from build123d import *

# Parameters (mm, degrees)
BOX001_W               = 20
BOX001_H               = 7.071068
BOX001_DEPTH           = 7.071068
BOX001_PLACEMENT_ANGLE = 45
BOX_W                  = 20
BOX_H                  = 10
BOX_DEPTH              = 10


with BuildPart() as cube001:
    # Box001 → Box001 (new body)
    with BuildSketch(Plane.XY):
        with Locations((10, 3.535534)):
            Rectangle(BOX001_W, BOX001_H)
    extrude(amount=BOX001_DEPTH)


with BuildPart() as cube001_1:
    # Box001 placement: moved
    add(cube001.part.moved(Location((0, 5, 5))).rotate(Axis((0, 5, 5), (1, 0, 0)), BOX001_PLACEMENT_ANGLE))


with BuildPart() as fusion:
    # Box → Box (new body)
    with BuildSketch(Plane.XY):
        with Locations((10, 5)):
            Rectangle(BOX_W, BOX_H)
    extrude(amount=BOX_DEPTH)

    # Fusion: union Cube001
    add(cube001_1.part)


solid = fusion.part
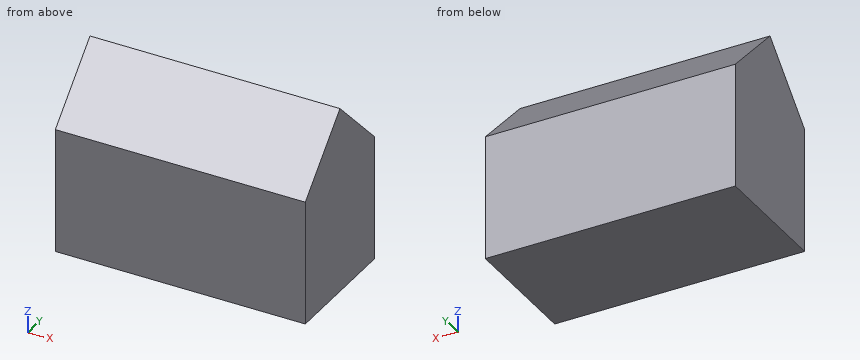
Work out the finished part from the listing and answer in its coordinate system (mm). Give positions to 0.01 mm unless a question says otherwise; leave off trailing zeros. Loops run counter-clockwise (first coordinate to the right, second up) from the corner with the lowest first, then second, coordinate; pieces in that order, holes last. Notation, with made-up numbers: (50.25, 7.25) - (57.25, 7.25) arc R4 ccw to (57.25, 14.25) - close; hole circle Ø7 at (-27, 59). An arc over 180 degrees is marked (long way). Answer in a Markdown table with one row per item. Add a question column.
Q1. The part is cut by section C-C (y = 1). Determine the outline of the cut face in (x, z).
Q2. Consider line 1 along Y through (x, z) = (18, 11.5); line 2 along Z through (x, y) = (12.5, 9); line 3 along Z through (x, y) = (9, 7). Determine where each line is inside the solid, lowest interval first.
Q3. The part is cut by section B-B (z = 11). Determine the outline of the cut face in (x, y), and give its area (3 significant figures).
Q4. This flat-tipped pin is pushed along its axis until it touches: P1, Ø1, axis at y = 3, z = 10, coming from the -X side. Where does it stop, or does it pass through?
Q5. The part is cut by section A-A (x = 7.25). Determine the outline of the cut face in (y, z), and give its area (3 significant figures).
Solution:
| question | item | result |
|---|---|---|
| 1 | outline | (0, 0) - (20, 0) - (20, 11) - (0, 11) - close |
| 2 | line 1 | y = 1.5 to 8.5 |
| 2 | line 2 | z = 0 to 11 |
| 2 | line 3 | z = 0 to 13 |
| 3 | outline | (0, 1) - (20, 1) - (20, 9) - (0, 9) - close |
| 3 | area | 160 mm² |
| 4 | P1 | stops at x = 0 |
| 5 | outline | (0, 0) - (10, 0) - (10, 10) - (5, 15) - (0, 10) - close |
| 5 | area | 125 mm² |
